```python
from build123d import *

# Parameters (mm, degrees)
SKETCH1_W           = 37
SKETCH1_H           = 11.7
BOSS_EXTRUDE1_DEPTH = 69
CUT_EXTRUDE1_DEPTH  = 67
SKETCH3_W           = 20
SKETCH3_H           = 5.9
CUT_EXTRUDE2_DEPTH  = 67
SKETCH5_R           = 1.9
BOSS_EXTRUDE3_DEPTH = 2
SKETCH7_R           = 1.9
BOSS_EXTRUDE4_DEPTH = 2
SKETCH8_W           = 3.5
SKETCH8_H           = 9
CUT_EXTRUDE3_DEPTH  = 40
BOSS_EXTRUDE5_START = 0.5
BOSS_EXTRUDE5_DEPTH = 2.5


with BuildPart() as part:
    # Sketch1 → Boss-Extrude1 (new body)
    with BuildSketch(Plane(origin=(0, 0, 0), x_dir=(1, 0, 0), z_dir=(0, 1, 0))):
        with Locations((18.5, 5.85)):
            Rectangle(SKETCH1_W, SKETCH1_H)
    extrude(amount=BOSS_EXTRUDE1_DEPTH)

    # Sketch2 → Cut-Extrude1 (cut)
    with BuildSketch(Plane(origin=(0, 69, 0), x_dir=(1, 0, 0), z_dir=(0, 1, 0))):
        Polygon((3, 0), (3, 2), (2, 2), (2, 3.8), (3, 3.8), (3, 9.7), (34, 9.7), (34, 3.8), (35, 3.8), (35, 2), (34, 2), (34, 0), align=None)
    extrude(amount=-CUT_EXTRUDE1_DEPTH, mode=Mode.SUBTRACT)

    # Sketch3 → Cut-Extrude2 (cut)
    with BuildSketch(Plane(origin=(0, 2, 0), x_dir=(1, 0, 0), z_dir=(0, 1, 0))):
        with Locations((19.275, 6.75)):
            Rectangle(SKETCH3_W, SKETCH3_H)
    extrude(amount=-CUT_EXTRUDE2_DEPTH, mode=Mode.SUBTRACT)

    # Sketch5 → Boss-Extrude3 (add)
    with BuildSketch(Plane(origin=(0, 0, -11.7), x_dir=(-1, 0, 0), z_dir=(0, 0, -1))):
        with BuildLine():
            Line((-14.12, 74.05), (-14.12, 69))
            Line((-14.12, 69), (-6.72, 69))
            Line((-6.72, 69), (-6.72, 74.05))
            ThreePointArc((-6.72, 74.05), (-10.42, 77.75), (-14.12, 74.05))
        make_face()
        with Locations((-10.42, 74.05)):
            Circle(SKETCH5_R, mode=Mode.SUBTRACT)
    extrude(amount=-BOSS_EXTRUDE3_DEPTH)

    # Sketch7 → Boss-Extrude4 (add)
    with BuildSketch(Plane.ZY):
        with BuildLine():
            Line((1.9, 87.05), (1.9, 79.55))
            ThreePointArc((1.9, 79.55), (1.65434509, 78.224292642), (0.95, 77.074621241))
            ThreePointArc((0.95, 77.074621241), (0.24565491, 75.924949841), (0, 74.599242482))
            Line((0, 74.599242482), (0, 69))
            Line((0, 69), (-11.7, 69))
            ThreePointArc((-11.7, 69), (-10.768790899, 74.577512686), (-8.076177285, 79.55))
            ThreePointArc((-8.076177285, 79.55), (-6.161996991, 83.084943588), (-5.5, 87.05))
            ThreePointArc((-5.5, 87.05), (-1.8, 90.75), (1.9, 87.05))
        make_face()
        with Locations((-1.8, 79.55)):
            Circle(SKETCH7_R, mode=Mode.SUBTRACT)
        with Locations((-1.8, 87.05)):
            Circle(SKETCH7_R, mode=Mode.SUBTRACT)
    extrude(amount=-BOSS_EXTRUDE4_DEPTH)

    # Sketch8 → Cut-Extrude3 (cut)
    with BuildSketch(Plane(origin=(37, 0, 0), x_dir=(0, 0, -1), z_dir=(1, 0, 0))):
        with Locations((3.25, 6.5)):
            Rectangle(SKETCH8_W, SKETCH8_H)
    extrude(amount=-CUT_EXTRUDE3_DEPTH, mode=Mode.SUBTRACT)

    # Sketch9 → Boss-Extrude5 (add)
    with BuildSketch(Plane.XY.offset(-5).offset(BOSS_EXTRUDE5_START)):
        with BuildLine():
            Line((37, 2), (37, 9.5))
            Line((37, 9.5), (35.75, 9.5))
            ThreePointArc((35.75, 9.5), (34.689339828, 9.060660172), (34.25, 8))
            Line((34.25, 8), (34.25, 7.5))
            ThreePointArc((34.25, 7.5), (34.542893219, 6.792893219), (35.25, 6.5))
            Line((35.25, 6.5), (35.25, 2))
            Line((35.25, 2), (37, 2))
        make_face()
    boss_extrude5 = extrude(amount=BOSS_EXTRUDE5_DEPTH)

    # Mirror1: Boss-Extrude5 across plane
    add(boss_extrude5.mirror(Plane(origin=(18.5, 0, 0), x_dir=(0, 0, 1), z_dir=(1, 0, 0))))


solid = part.part
```
Input: part model. Units: mm. Frame: model coordinates. A direction names the side the tool comes from. Give positions to 0.01 mm unless a question says otherwise; leave off trailing zeros. Order: outer loops, then holes, each group sorted by start corner. A loop starts at its lowest first (then second) coordinate and runs counter-clockwise, first axis right, second up. Notation, with made-up numbers: M 15.5,-28.75 L 49.5,-28.75 A27 cw 49.5,3.25 Z; hole C 54,61.25 d9. An arc over 180 degrees is marked long. Return JSON: item names as keys, results as strings.
1) Mould query, pull axis X, two halves, no side actions, for faces 1 (the face through (2, 66, -3)), 2 (the face through (0, 46, -5)), 3 (the face through (2, 29, 0)). Classes: released by +X, released by -X, zero draft, split by the parting line, or undercut.
Taken from the geometry:
{"face 1": "undercut", "face 2": "released by -X", "face 3": "zero draft"}
2) Line query: L1, parallel to Y at x = 0.45, z = -1.8; L2, parallel to X at y = 74.05, z = -10.25; L3, parallel to X at y = 14.5, z = -2.5. Output: solid intervals per line, ascending. Write a range as [from, to].
Taken from the geometry:
{"L1": "y = [0, 2], [11, 77.65], [81.45, 85.15], [88.95, 90.75]", "L2": "x = [0, 2], [6.72, 8.52], [12.32, 14.12]", "L3": "x = [0, 2], [35, 37]"}
3) Section query B-B on y = 63. Output: boundary loops of the cut face in (x, z), and give its area (3 significant figures).
Taken from the geometry:
{"outline": "M 0,-11.7 L 37,-11.7 L 37,0 L 34,0 L 34,-2 L 35,-2 L 35,-3.8 L 34,-3.8 L 34,-9.7 L 3,-9.7 L 3,-3.8 L 2,-3.8 L 2,-2 L 3,-2 L 3,0 L 0,0 Z", "area": "129 mm2"}
4) Access query for faces 4 (the face through (34, 36, -7)), 5 (the face through (36, 6, -1.5)), 6 (the face through (2.3, 9.07, -3.27)). Directions: +Z, -Z, +X, -X, +Y, -Y. A direction counts if a zero-diameter tool reaches every point of the face in a straight line with its end or side. Return the directions, or none.
Taken from the geometry:
{"face 4": "+Z, +Y", "face 5": "+X, -X", "face 6": "none"}
5) Section query C-C on x = 10.42. Output: boundary loops of the cut face in (y, z), and give its area (4 significant figures).
Taken from the geometry:
{"outline": "M 0,-11.7 L 72.15,-11.7 L 72.15,-9.7 L 0,-9.7 Z; M 0,-3.8 L 2,-3.8 L 2,0 L 0,0 Z; M 75.95,-11.7 L 77.75,-11.7 L 77.75,-9.7 L 75.95,-9.7 Z", "area": "155.5 mm2"}
6) Contact query for flat-ended pins moving along their axis: pin 1 (8 mm diameter, centred on x = 7.5, y = 35, fed in from +Z); pin 2 (3.5 mm diameter, centred on x = 36, z = -2.5, fed in from -Y); pin 3 (1.4 mm diameter, centred on x = 36.5, z = -4, fed in from +Y); pin 4 (2 mm diameter, centred on x = 35.5, y = 6.5, fed in from +Z). Output: stop coordinate, or through.
Taken from the geometry:
{"pin 1": "stops at z = -9.7", "pin 2": "stops at y = 0", "pin 3": "stops at y = 69", "pin 4": "stops at z = 0"}
7) Section query D-D on x = 31. Output: boundary loops of the cut face in (y, z).
Taken from the geometry:
{"outline": "M 0,-11.7 L 69,-11.7 L 69,-9.7 L 2,-9.7 L 2,0 L 0,0 Z"}
8) Section query A-A on x = 15. Output: boundary loops of the cut face in (y, z), and give its area (3 significant figures).
Taken from the geometry:
{"outline": "M 0,-11.7 L 69,-11.7 L 69,-9.7 L 0,-9.7 Z; M 0,-3.8 L 2,-3.8 L 2,0 L 0,0 Z", "area": "146 mm2"}
